from build123d import *

# Parameters (mm, degrees)
SKETCH008_R     = 35.5
PAD007_DEPTH    = 30
SKETCH009_R     = 24
POCKET001_DEPTH = 25
SKETCH010_R     = 8
PAD008_DEPTH    = 16
POCKET002_DEPTH = 2.5
SKETCH012_R     = 1.5
POCKET003_DEPTH = 25
FILLET_R        = 3
FILLET001_R     = 3


with BuildPart() as part:
    # Sketch008 → Pad007 (new body)
    with BuildSketch(Plane.YZ):
        with Locations((-2.086398, 2.086246)):
            Circle(SKETCH008_R)
    extrude(amount=PAD007_DEPTH)

    # Sketch009 (on Face2 of Pad007) → Pocket001 (cut)
    with BuildSketch(Plane(origin=(0, 0, 0), x_dir=(0, 1, 0), z_dir=(-1, 0, 0))):
        with Locations((-1.664763, -2.119737)):
            Circle(SKETCH009_R)
    extrude(amount=-POCKET001_DEPTH, mode=Mode.SUBTRACT)

    # Sketch010 (on Face5 of Pocket001) → Pad008 (join)
    with BuildSketch(Plane(origin=(25, 0, 0), x_dir=(0, 1, 0), z_dir=(-1, 0, 0))):
        with Locations((-1.350817, -2.732668)):
            Circle(SKETCH010_R)
    extrude(amount=PAD008_DEPTH)

    # Sketch011 (on Face7 of Pad008) → Pocket002 (cut)
    with BuildSketch(Plane(origin=(9, 0, 0), x_dir=(0, 1, 0), z_dir=(-1, 0, 0))):
        Polygon((-1.111872, 4.248012), (-7.222761, 0.700721), (-7.206161, -6.365109), (-1.078672, -9.883648), (5.032216, -6.336357), (5.015616, 0.729474), align=None)
    extrude(amount=-POCKET002_DEPTH, mode=Mode.SUBTRACT)

    # Sketch012 (on Face14 of Pocket002) → Pocket003 (cut)
    with BuildSketch(Plane(origin=(11.5, 0, 0), x_dir=(0, 1, 0), z_dir=(-1, 0, 0))):
        with Locations((-0.927213, -2.793039)):
            Circle(SKETCH012_R)
    extrude(amount=-POCKET003_DEPTH, mode=Mode.SUBTRACT)

    # Fillet
    fillet_edges = [part.edges().sort_by_distance(p)[0] for p in [
        (0, -37.586398, 2.086246),
    ]]
    fillet(fillet_edges, radius=FILLET_R)

    # Fillet001
    fillet001_edges = [part.edges().sort_by_distance(p)[0] for p in [
        (30, -37.586398, 2.086246),
    ]]
    fillet(fillet001_edges, radius=FILLET001_R)


with BuildPart() as part_1:
    # Body003 placement: moved
    add(part.part.moved(Location((55, -37, 20))))


solid = part_1.part
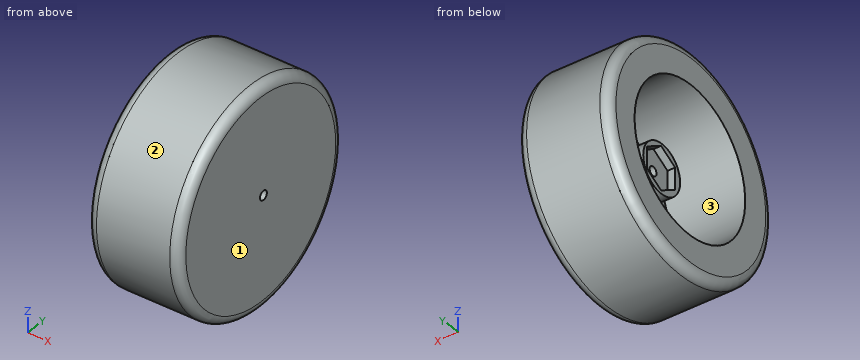
Geometry: final body of the model. Coordinates: model frame, mm. Face numbers are marked on the shaded views. Give positions to 0.01 mm unless a question says otherwise; leave off trailing zeros. Loops run counter-clockwise (first coordinate to the right, second up) from the corner with the lowest first, then second, coordinate; pieces in that order, holes last. Notation, with made-up numbers: M 34.5,5 L 61.5,5 A15 ccw 61.5,11 Z; hole C 66.5,56 d7. An arc over 180 degrees is marked long. Put each result on its own line as item: value.
1) Cut plane B-B, the plane x = 81. Return the cut outline in (y, z).
Computed values:
outline: C -39.09,22.09 d71; hole C -37.93,22.79 d3
2) First-contact query: P1, Ø3, axis at x = 76, y = -45.5, coming from the +Z side; P2, Ø10, axis at x = 73, z = 42, coming from the -Y side; P3, Ø4, axis at x = 69.5, z = 1, coming from the +Y side. Flat tips, straight axial feed; report the tip coordinate or a pass-through.
Computed values:
P1: stops at z = 57.24
P2: stops at y = -71.3
P3: stops at y = -9.15
3) Mould query, pull axis Y, two halves, no side actions, for the marked faces 1, 2 and 3. Classes: released by +Y, released by -Y, zero draft, split by the parting line, or undercut.
Computed values:
face 1: zero draft
face 2: split by the parting line
face 3: undercut
4) Cut plane A-A, the plane x = 71.75. Return the cut outline in (y, z).
Computed values:
outline: C -39.09,22.09 d71; C -38.35,22.73 d16; hole C -38.66,22.12 d48; hole C -37.93,22.79 d3
5) Cut plane C-C, the plane x = 57. Return the cut outline in (y, z), plus the area to 3 significant figures.
Computed values:
outline: C -39.09,22.09 d70.66; hole C -38.66,22.12 d48
area: 2,110 mm^2
6) Material intervals for L1, parallel to Y at x = 72.25, z = 22.5; L2, parallel to Z at x = 64.5, y = -45.5; L3, parallel to Y at x = 71.75, z = 22, sorted ascending. Write a range as from..to.
Computed values:
L1: y = -74.58..-62.66, -46.35..-39.4, -36.46..-30.35, -14.67..-3.59
L2: z = -12.83..-0.89, 19.14..26.32, 45.13..57
L3: y = -74.59..-62.66, -46.32..-39.2, -36.65..-30.38, -14.67..-3.59
